Source: CAD feature listing. Evaluate the final solid. Frame: model axes, mm. A direction names the side the tool comes from. Round coordinates to 2 decimals unless told otherwise and drop trailing zeros. Order: outer loops, then holes, each group sorted by start corner. A loop starts at its lowest first (then second) coordinate and runs counter-clockwise, first axis right, second up. Notation, with made-up numbers: (52.25, -34.5) - (98.25, -34.5) arc R24 ccw to (98.25, -12.5) - close; hole circle Ø7 at (60, 33). An arc over 180 degrees is marked (long way). Put each result on its own line as item: value. Start each with the question number.
1) Access query for faces 1 (the face through (-0.59, -14.51, -4.46)), 2 (the face through (0, 52.1, 3)). Directions: +Z, -Z, +X, -X, +Y, -Y. A direction counts if a zero-diameter tool reaches every point of the face in a straight line with its end or side. Return the directions, or none.
2) Section C-C on z = 0. Output: boundary loops of the cut face in (x, y).
3) Mould query, pull axis Y, two halves, no side actions, for faces 3 (the face through (-0.585, 18.79, 2.636)), 4 (the face through (0, 53.9, 0)), 5 (the face through (-0.59, 52.99, -4.46)). Classes: +Y half, -Y half, draft (parallel to the pull), parting line (faces both ways), or undercut.
4) Section A-A on z = -3.5. Output: boundary loops of the cut face in (x, y), then the cut area to 3 significant figures.
5) Section D-D on y = -2.5. Output: boundary loops of the cut face in (x, z).
6) Line query: probe 1 along Y at (x, z) = (-0.25, 4); probe 2 along X at (y, z) = (40, -0.25); probe 3 along Z at (x, y) = (-1, -5.5). Output: solid intervals per line, ascending. Write a range as [from, to].
7) Contact query for flat-ended pins moving along their axis: P1, Ø2, axis at y = 20, z = -2, coming from the -X side; P2, Ø1.5, axis at x = 0.5, y = 45.5, coming from the -Z side; P3, Ø1.5, axis at y = 1, z = 0, coming from the +X side. Output: stop coordinate, or through.
8) Section B-B on x = 0. Output: boundary loops of the cut face in (y, z).
```python
from build123d import *

# Parameters (mm, degrees)
SKETCH1_R           = 2.5
BOSS_EXTRUDE1_DEPTH = 1
SKETCH2_R           = 1.5
BOSS_EXTRUDE2_DEPTH = 36.5
SKETCH3_R           = 2.5
BOSS_EXTRUDE3_DEPTH = 1
SCALE1_SCALE        = 1.8


with BuildPart() as part:
    # Sketch1 → Boss-Extrude1 (new body)
    with BuildSketch(Plane(origin=(0, 0, 0), x_dir=(1, 0, 0), z_dir=(0, 1, 0))):
        Circle(SKETCH1_R)
    extrude(amount=BOSS_EXTRUDE1_DEPTH)

    # Sketch2 → Boss-Extrude2 (add)
    with BuildSketch(Plane(origin=(0, 1, 0), x_dir=(1, 0, 0), z_dir=(0, 1, 0))):
        Circle(SKETCH2_R)
    extrude(amount=BOSS_EXTRUDE2_DEPTH)

    # Sketch3 → Boss-Extrude3 (add)
    with BuildSketch(Plane(origin=(0, 37.5, 0), x_dir=(1, 0, 0), z_dir=(0, 1, 0))):
        Circle(SKETCH3_R)
    extrude(amount=BOSS_EXTRUDE3_DEPTH)


with BuildPart() as part_1:
    # Scale1: scaled about (0, 19.25, 0)
    add(part.part.scale(SCALE1_SCALE).moved(Location((0, -15.4, 0))))


solid = part_1.part
```
Answer sheet:
1. face 1: +Y, -Y
1. face 2: none
2. outline: (-4.5, -15.4) - (4.5, -15.4) - (4.5, -13.6) - (2.7, -13.6) - (2.7, 52.1) - (4.5, 52.1) - (4.5, 53.9) - (-4.5, 53.9) - (-4.5, 52.1) - (-2.7, 52.1) - (-2.7, -13.6) - (-4.5, -13.6) - close
3. face 3: undercut
3. face 4: +Y half
3. face 5: draft
4. outline: (-2.83, -15.4) - (2.83, -15.4) - (2.83, -13.6) - (-2.83, -13.6) - close; (-2.83, 52.1) - (2.83, 52.1) - (2.83, 53.9) - (-2.83, 53.9) - close
4. area: 20.4 mm^2
5. outline: circle Ø5.4 at (0, 0)
6. probe 1: [-15.4, -13.6], [52.1, 53.9]
6. probe 2: [-2.69, 2.69]
6. probe 3: [-2.51, 2.51]
7. P1: x = -2.51
7. P2: z = -2.7
7. P3: x = 2.7
8. outline: (-15.4, -4.5) - (-13.6, -4.5) - (-13.6, -2.7) - (52.1, -2.7) - (52.1, -4.5) - (53.9, -4.5) - (53.9, 4.5) - (52.1, 4.5) - (52.1, 2.7) - (-13.6, 2.7) - (-13.6, 4.5) - (-15.4, 4.5) - close
